The listing builds one solid part. Answer for the finished solid, in the listing's coordinates (mm). A direction names the side the tool comes from. Coordinates: 2 decimals unless noted, no trailing zeros. Order: outer loops, then holes, each group sorted by start corner. A loop starts at its lowest first (then second) coordinate and runs counter-clockwise, first axis right, second up. Notation, with made-up numbers: (58.5, 37.25) - (87.5, 37.25) arc R27 ccw to (87.5, 70.25) - close; hole circle Ø8 at (47, 16). An arc over 180 degrees is marked (long way). One line per item, written item: value. Start each with the question number.
```python
from build123d import *

# Parameters (mm, degrees)
SKETCH5_R          = 0.5
CUT_EXTRUDE1_DEPTH = 10
SKETCH6_W          = 703.629675086
SKETCH6_H          = 157.863240862
CUT_EXTRUDE2_DEPTH = 90


with BuildPart() as part:
    # Sketch1 → Revolve1 (revolve)
    with BuildSketch(Plane.XY):
        Polygon((-315, 2), (-315, 37), (135, 37), (184.985180236, 2), (194.985180236, 2), (194.985180236, 0), (-125, 0), (-325, 0), (-325, 2), align=None)
    revolve(axis=Axis((-125, 0, 0), (1, 0, 0)))


with BuildPart() as body_2:
    # Sketch4 → Revolve2 (revolve)
    with BuildSketch(Plane(origin=(0, 0, 0), x_dir=(1, 0, 0), z_dir=(0, 1, 0))):
        Polygon((23, 0), (23, 10), (13.172803675, 37), (10.172803675, 37), (20, 10), (20, 0), align=None)
    revolve(axis=Axis((20, 0, 0), (1, 0, 0)))

    # Sketch5 → Cut-Extrude1 (cut)
    with BuildSketch(Plane.ZY.offset(-20)):
        Circle(SKETCH5_R)
    extrude(amount=-CUT_EXTRUDE1_DEPTH, mode=Mode.SUBTRACT)


with BuildPart() as part_1:
    add(part.part)

    # Combine1: cut body 2
    add(body_2.part, mode=Mode.SUBTRACT)

    # Sketch6 → Cut-Extrude2 (cut)
    with BuildSketch(Plane.XY):
        Rectangle(SKETCH6_W, SKETCH6_H)
    extrude(amount=-CUT_EXTRUDE2_DEPTH, mode=Mode.SUBTRACT)


solid = part_1.part
```
(1) Flat-ended cylindrical pins translate along their axes: pin 1 Ø6 at (x, z) = (-230, 23) entering from -Y; pin 2 Ø3 at (y, z) = (-2.5, 5.5) entering from +X; pin 3 Ø2 at (y, z) = (-22, 15) entering from -X. Find the tip coordinate at first contact, or state that the pin passes through.
(2) For faces 1 (the face through (74.94, 0.81, 36.99)), 2 (the face through (23, 0, 4)), determine the directions among +Z, -Z, +X, -X, +Y, -Y from which every point of the face is accessible in a straight line to the end or side of a thin tool.
(3) For a pull along Z with two mould halves and no side action, classify faces 3 (the face through (-150.14, 0.81, 36.99)), 4 (the face through (21.29, 0.32, 14.69)), 5 (the face through (-315, 1, 15)), 6 (the face through (-69, 1, 0)) as pulls with the +Z half, pulls with the -Z half, needs draft (parallel to the pull), parting line crosses it, or undercut.
(4) The part is cut by section A-A on x = -64. Determine the outline of the cut face in (y, z), plus the area to 3 significant figures.
(5) Consider probe 1 along X at (y, z) = (-19.5, 10); probe 2 along X at (y, z) = (-9.5, 8); probe 3 along Y at (x, z) = (-269.5, 14). Determine where each line is inside the solid, lowest interval first.
Completed:
1. pin 1: stops at y = -31.13
1. pin 2: stops at x = 181.36
1. pin 3: stops at x = -315
2. face 1: +Z, +X, -X
2. face 2: none
3. face 3: pulls with the +Z half
3. face 4: undercut
3. face 5: needs draft
3. face 6: pulls with the -Z half
4. outline: (-37, 0) - (37, 0) arc R37 ccw to start
4. area: 2,150 mm2
5. probe 1: x = -315 to 15.66, 18.66 to 156.54
5. probe 2: x = -315 to 19.12, 22.12 to 170.1
5. probe 3: y = -34.25 to 34.25
